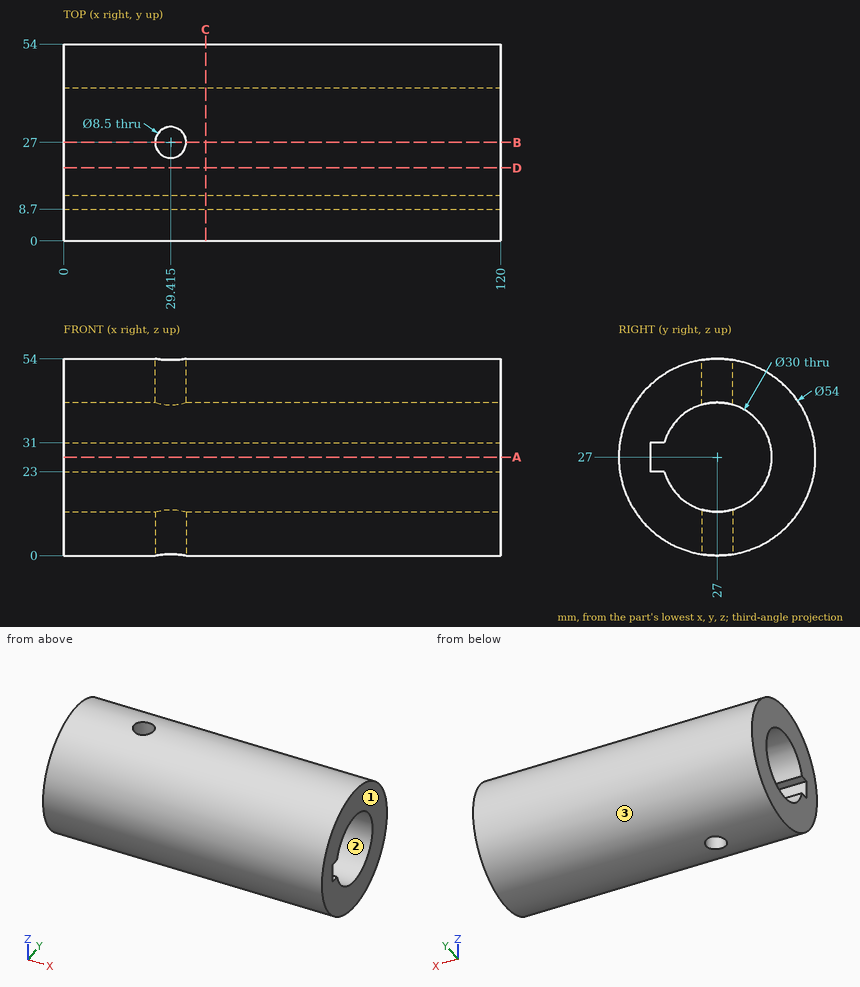
Geometry: see drawing. Coordinates: mm, zero at the bounding-box minimum. Coordinates: 2 decimals unless noted, no trailing zeros. Loops run counter-clockwise (first coordinate to the right, second up) from the corner with the lowest first, then second, coordinate; pieces in that order, holes last. Notation, with made-up numbers: (25.25, 64) - (69.25, 64) arc R28 ccw to (69.25, 102) - close; hole circle Ø9 at (-21.5, 69.25). An arc over 180 degrees is marked (long way). Answer in a Markdown table with one row per item.
(1) Mould query, pull axis Y, two halves, no side actions, for the marked faces 1, 2 and 3. Classes: pulls with the +Y half, pulls with the -Y half, needs draft (parallel to the pull), parting line crosses it, or undercut.
Model answer:
| item | result |
|---|---|
| face 1 | needs draft |
| face 2 | undercut |
| face 3 | parting line crosses it |
(2) Cut plane B-B on y = 27. Output: boundary loops of the cut face in (x, z) (3 decimals).
Model answer:
| item | result |
|---|---|
| outline | (0, 0) - (25.165, 0) - (25.165, 12) - (0, 12) - close; (0, 42) - (25.165, 42) - (25.165, 54) - (0, 54) - close; (33.665, 0) - (120, 0) - (120, 12) - (33.665, 12) - close; (33.665, 42) - (120, 42) - (120, 54) - (33.665, 54) - close |
(3) Pin query (flat end, axial travel): P1, Ø1.5, axis at x = 94, y = 45, coming from the -Z side; P2, Ø1.2, axis at x = 51.5, y = 11, coming from the +Z side; P3, Ø5, axis at x = 53, y = 24, coming from the -Z side. Return the tip coordinate at first contact, or that it passes through.
Model answer:
| item | result |
|---|---|
| P1 | stops at z = 6.23 |
| P2 | stops at z = 49.18 |
| P3 | stops at z = 0 |
(4) Cut plane C-C on x = 39. Output: boundary loops of the cut face in (y, z).
Model answer:
| item | result |
|---|---|
| outline | circle Ø54 at (27, 27); hole (8.7, 23) - (12.54, 23) arc R15 ccw (long way) to (12.54, 31) - (8.7, 31) - close |
(5) Cut plane A-A on z = 27. Output: boundary loops of the cut face in (x, y), plus the area to 3 significant figures.
Model answer:
| item | result |
|---|---|
| outline | (0, 0) - (120, 0) - (120, 8.7) - (0, 8.7) - close; (0, 42) - (120, 42) - (120, 54) - (0, 54) - close |
| area | 2,480 mm² |
(6) Cut plane D-D on y = 20. Output: boundary loops of the cut face in (x, z).
Model answer:
| item | result |
|---|---|
| outline | (0, 0.92) - (120, 0.92) - (120, 13.73) - (0, 13.73) - close; (0, 40.27) - (120, 40.27) - (120, 53.08) - (0, 53.08) - close |
(7) Material intervals for L1, parallel to X at y = 27, z = 50.5 (3 decimals); L2, parallel to Z at x = 60.5, y = 27; L3, parallel to Y at x = 12, z = 32.5 (1 decimal), sorted ascending. Write a range as from..to.
Model answer:
| item | result |
|---|---|
| L1 | x = 0..25.165, 33.665..120 |
| L2 | z = 0..12, 42..54 |
| L3 | y = 0.6..13, 41..53.4 |
